from build123d import *

# Parameters (mm, degrees)
SKETCH_1_W          = 8
SKETCH_1_H          = 10
EXTRUDE_1_DEPTH     = 3
EXTRUDE_2_DEPTH     = 10
SKETCH_3_R          = 2.5
CUT_EXTRUDE_1_DEPTH = 10
SKETCH_4_W          = 2.082831863
SKETCH_4_H          = 7.092942697
EXTRUDE_3_DEPTH     = 0.1


with BuildPart() as part:
    # 草图1 → 凸台-拉伸1 (new body)
    with BuildSketch(Plane(origin=(0, 0, 0), x_dir=(1, 0, 0), z_dir=(0, 1, 0))):
        with Locations((4, 5)):
            Rectangle(SKETCH_1_W, SKETCH_1_H)
    extrude(amount=EXTRUDE_1_DEPTH)

    # 草图2 → 凸台-拉伸2 (add)
    with BuildSketch(Plane(origin=(0, 3, 0), x_dir=(1, 0, 0), z_dir=(0, 1, 0))):
        with BuildLine():
            Line((0.005966473, 5), (0, 0))
            Line((0, 0), (8, 0))
            Line((8, 0), (7.994033527, 5))
            ThreePointArc((7.994033527, 5), (4, 8.994033527), (0.005966473, 5))
        make_face()
    extrude(amount=EXTRUDE_2_DEPTH)

    # 草图3 → 切除-拉伸1 (cut)
    with BuildSketch(Plane.XZ):
        with Locations(Location((4, -5.512337614, 0), (0, 0, 270))):
            Circle(SKETCH_3_R)
    extrude(amount=-CUT_EXTRUDE_1_DEPTH, mode=Mode.SUBTRACT)

    # 草图4 → 凸台-拉伸3 (add)
    with BuildSketch(Plane(origin=(0, 13, 0), x_dir=(1, 0, 0), z_dir=(0, 1, 0))):
        with Locations((4.131440846, 3.546471349)):
            Rectangle(SKETCH_4_W, SKETCH_4_H)
    extrude(amount=EXTRUDE_3_DEPTH)


solid = part.part
Source: CAD feature listing. Evaluate the final solid. Frame: model axes, mm. A direction names the side the tool comes from. Coordinates: 2 decimals unless noted, no trailing zeros. Loops run counter-clockwise (first coordinate to the right, second up) from the corner with the lowest first, then second, coordinate; pieces in that order, holes last. Notation, with made-up numbers: M 47,11.5 L 88,11.5 A30 ccw 88,38.5 Z; hole C 32,20.5 d1. An arc over 180 degrees is marked long. Answer in a Markdown table with one row per item.
Q1. Section B-B on x = 5. Return the cut outline in (y, z), plus the area to 3 significant figures.
Answers below:
| item | result |
|---|---|
| outline | M 0,-10 L 3,-10 L 3,-8.87 L 13,-8.87 L 13,-7.09 L 13.1,-7.09 L 13.1,0 L 0,0 L 0,-3.22 L 10,-3.22 L 10,-7.8 L 0,-7.8 Z |
| area | 73.6 mm^2 |
Q2. Section A-A on y = 8.25. Return the cut outline in (x, z), plus the area to 3 significant figures.
Answers below:
| item | result |
|---|---|
| outline | M 0,0 L 0.01,-5 A3.99 ccw 7.99,-5 L 8,0 Z; hole C 4,-5.51 d5 |
| area | 45.4 mm^2 |
Q3. First-contact query: pin 1 (3 mm diameter, centred on x = 5.5, y = 6, fed in from -Z); pin 2 (6 mm diameter, centred on y = 11, z = -7.5, fed in from -X). Flat tips, straight axial feed; report the tip coordinate or a pass-through.
Answers below:
| item | result |
|---|---|
| pin 1 | stops at z = -8.99 |
| pin 2 | stops at x = 0.01 |
Q4. Ray query, probe 1 along Y at (x, z) = (2.5, -5); probe 2 along Y at (x, z) = (7.5, -3); probe 3 along X at (y, z) = (12.5, -1.5). Return the intervals inside material, ascending. Write a range as from..to.
Answers below:
| item | result |
|---|---|
| probe 1 | y = 10..13 |
| probe 2 | y = 0..13 |
| probe 3 | x = 0..8 |
Q5. Draft query along X for faces 3 (the cylindrical face through (4.751, 4.93, -7.897)), 4 (the flat face through (4, 10, -5)), 5 (the flat face through (0, 1, -5)), 6 (the flat face through (4, 3, -9.5)). Return one class per face: pulls with the +X half, pulls with the -X half, needs draft (parallel to the pull), parting line crosses it, or undercut.
Answers below:
| item | result |
|---|---|
| face 3 | undercut |
| face 4 | undercut |
| face 5 | pulls with the -X half |
| face 6 | needs draft |
Q6. Section C-C on y = 12. Return the cut outline in (x, z), plus the area to 3 significant figures.
Answers below:
| item | result |
|---|---|
| outline | M 0,0 L 0.01,-5 A3.99 ccw 7.99,-5 L 8,0 Z |
| area | 65.0 mm^2 |
Q7. Set-up query: faces 1 (the flat face through (4, 1, -10)), 2 (the cylindrical face through (4.088, 7.93, -8.993)). Return all of +Z, -Z, +X, -X, +Y, -Y with unobstructed straight access to the full face (end or side cutting, diameter ignored); none if empty.
Answers below:
| item | result |
|---|---|
| face 1 | -Z, +X, -X, +Y, -Y |
| face 2 | -Z, +Y |
